Check sheet for the modelled part. Datum: model origin and axes. Units: mm. A direction names the side the tool comes from. Coordinates: 2 decimals unless noted, no trailing zeros. Loops run counter-clockwise (first coordinate to the right, second up) from the corner with the lowest first, then second, coordinate; pieces in that order, holes last. Notation, with made-up numbers: (66, 2) -> (112, 2) arc R14 ccw to (112, 24) -> close; hole circle Ø8 at (45.25, -37.75). An arc over 180 degrees is marked (long way). Use one line per item in the form item = value.
from build123d import *

# Parameters (mm, degrees)
SKETCH1_W           = 25.4
SKETCH1_H           = 25.4
SKETCH1_W_2         = 22.4
SKETCH1_H_2         = 22.4
BOSS_EXTRUDE1_DEPTH = 355
CUT_EXTRUDE2_DEPTH  = 25.4


with BuildPart() as part:
    # Sketch1 → Boss-Extrude1 (new body)
    with BuildSketch(Plane.XY):
        Rectangle(SKETCH1_W, SKETCH1_H)
        Rectangle(SKETCH1_W_2, SKETCH1_H_2, mode=Mode.SUBTRACT)
    extrude(amount=BOSS_EXTRUDE1_DEPTH)

    # Sketch3 → Cut-Extrude2 (cut)
    with BuildSketch(Plane.ZY.offset(12.7)):
        Polygon((0, -12.7), (23.62, 12.7), (0, 12.7), align=None)
    extrude(amount=-CUT_EXTRUDE2_DEPTH, mode=Mode.SUBTRACT)


solid = part.part
(1) Mould release check, pull along X, two halves, no side actions. Record for faces 3 (the flat face through (-11.35, 0.06, 355)), 4 (the flat face through (12.7, 0, 175)), 5 (the flat face through (-11.2, 0, 176)): +X half, -X half, draft (parallel to the pull), parting line (faces both ways), or undercut.
Established:
face_3 = draft
face_4 = +X half
face_5 = undercut
(2) Section check C-C, the plane y = 1.5. Record the boundary of the cut face in (x, z).
Established:
outline = (-12.7, 13.2) -> (-11.2, 13.2) -> (-11.2, 355) -> (-12.7, 355) -> close; (11.2, 13.2) -> (12.7, 13.2) -> (12.7, 355) -> (11.2, 355) -> close
(3) Section check A-A, the plane x = -6.5. Record the boundary of the cut face in (y, z).
Established:
outline = (-12.7, 0) -> (-11.2, 1.39) -> (-11.2, 355) -> (-12.7, 355) -> close; (11.2, 22.23) -> (12.7, 23.62) -> (12.7, 355) -> (11.2, 355) -> close
(4) Section check B-B, the plane z = 82.5. Record the boundary of the cut face in (x, y).
Established:
outline = (-12.7, -12.7) -> (12.7, -12.7) -> (12.7, 12.7) -> (-12.7, 12.7) -> close; hole (-11.2, -11.2) -> (11.2, -11.2) -> (11.2, 11.2) -> (-11.2, 11.2) -> close
(5) Go/stop test with a flat-tipped pin: P1, Ø5, axis at x = -8, y = 9, coming from the -Z side. Record where the tip stops, or that it passes through.
Established:
P1 = 22.23
(6) Tool access check on faces 1 (the flat face through (11.2, 0, 176)), 2 (the flat face through (0, -12.7, 175)). Record the directions out of +Z, -Z, +X, -X, +Y, -Y that give a thin tool (end or side, any length) a straight path to the whole face; none if there is none.
Established:
face_1 = +Z, -Z
face_2 = +Z, -Z, +X, -X, -Y
(7) Scan lines: line 1 along Y through (x, z) = (6.5, 172); line 2 along Y through (x, z) = (-9.5, 19). Record each from-to range of solid material in increasing order.
Established:
line_1 = -12.7 to -11.2, 11.2 to 12.7
line_2 = -12.7 to -11.2
